Here's how the part is built. I have some questions about the finished solid (model axes, mm). Round coordinates to 2 decimals unless told otherwise and drop trailing zeros. Loops run counter-clockwise (first coordinate to the right, second up) from the corner with the lowest first, then second, coordinate; pieces in that order, holes last. Notation, with made-up numbers: (-39.5, 40.25) - (8.5, 40.25) arc R13 cw to (8.5, 54.25) - close; hole circle Ø5 at (34, -38). An arc over 180 degrees is marked (long way). Answer as a JSON object with one key per item and string values. Group by question number.
1) If I drill on line 1 along Y through (x, z) = (-1, 1.65); line 2 along X through (y, z) = (-53.5, 1.85); line 3 along X through (y, z) = (14.5, 0.5), over which ranges is the centre line in solid material (lowest first)? Write a range as [from, to].
2) I want a section at B-B, the plane x = 38. Please give me the cut outline in (y, z).
3) I want a section at C-C, the plane y = -53.5. Please give me the cut outline in (x, z).
4) I want a section at A-A, the plane z = 1.85. Please give me the cut outline in (x, y), then the cut area to 3 significant figures.
from build123d import *

# Parameters (mm, degrees)
F1_DEPTH    = 2.4268273264
F2_T1_DEPTH = 99.1532575298
F3_T1_DEPTH = 59.396472342
F4_T1_DEPTH = 59.396472342
F5_T1_DEPTH = 107.0840707021
F6_T1_DEPTH = 101.9910508867


# Not quite as in the source:
# - a fillet or chamfer that OpenCascade refuses, or shapes differently, is made with other operations: its cross-section is extruded or revolved along the edge and cut away or added


with BuildPart() as f1:
    # F0 (on Top) → F1 (new body)
    with BuildSketch(Plane.XY):
        Polygon((0, 32.5707793236), (-36.5124791861, 32.5707793236), (-58.7103962898, 0), (0, -63.0669593811), align=None)
        Polygon((36.5124791861, 32.5707793236), (0, 32.5707793236), (0, -63.0669593811), (58.7103962898, 0), align=None)
    extrude(amount=F1_DEPTH)

    # F2: chamfer of 5.08 on 1 edges, made by hand

    # F2_s2 → F2_t1 (cut)
    with BuildSketch(Plane.YZ.offset(-49.5766287649)):
        Polygon((32.5707793236, -2.6531726736), (27.4907793236, 2.4268273264), (32.5707793236, 2.4268273264), align=None)
    extrude(amount=F2_T1_DEPTH, mode=Mode.SUBTRACT)

    # F3: chamfer of 5.08 on 1 edges, made by hand

    # F3_s2 → F3_t1 (cut)
    with BuildSketch(Plane(origin=(7.4722902543, 10.964015938, 0), x_dir=(0, 0, 1), z_dir=(-0.5631734509, -0.8263387103, 0))):
        Polygon((-2.6531726736, 48.5146731522), (2.4268273264, 43.4346731522), (2.4268273264, 48.5146731522), align=None)
    extrude(amount=F3_T1_DEPTH, mode=Mode.SUBTRACT)

    # F4: chamfer of 5.08 on 1 edges, made by hand

    # F4_s2 → F4_t1 (cut)
    with BuildSketch(Plane(origin=(25.9782260477, -38.1175884143, 0), x_dir=(0, 0, 1), z_dir=(-0.5631734509, 0.8263387103, 0))):
        Polygon((-2.6531726736, 48.5146731522), (2.4268273264, 43.4346731522), (2.4268273264, 48.5146731522), align=None)
    extrude(amount=F4_T1_DEPTH, mode=Mode.SUBTRACT)

    # F5: chamfer of 5.08 on 1 edges, made by hand

    # F5_s2 → F5_t1 (cut)
    with BuildSketch(Plane(origin=(-40.354442867, -43.3489155239, 0), x_dir=(0, 0, 1), z_dir=(0.6813742779, 0.7319351703, 0))):
        Polygon((-2.6531726736, 42.9722039049), (2.4268273264, 37.8922039049), (2.4268273264, 42.9722039049), align=None)
    extrude(amount=F5_T1_DEPTH, mode=Mode.SUBTRACT)

    # F6: chamfer of 5.08 on 1 edges, made by hand

    # F6_s2 → F6_t1 (cut)
    with BuildSketch(Plane(origin=(-32.6098884775, 35.0296819984, 0), x_dir=(0, 0, 1), z_dir=(0.6813742779, -0.7319351703, 0))):
        Polygon((-2.6531726736, 42.9722039049), (2.4268273264, 37.8922039049), (2.4268273264, 42.9722039049), align=None)
    extrude(amount=F6_T1_DEPTH, mode=Mode.SUBTRACT)


solid = f1.part
Outcome:
{
 "1": {"line 1": "[-55.68, 28.27]", "line 2": "[-2.75, 2.75]", "line 3": "[-45.01, 45.01]"},
 "2": {"outline": "(-18.35, 0) - (25.68, 0) - (21.37, 2.43) - (-14.79, 2.43) - close"},
 "3": {"outline": "(-5.28, 0) - (5.28, 0) - (1.97, 2.43) - (-1.97, 2.43) - close"},
 "4": {"outline": "(-52.96, 0.44) - (0, -56.46) - (52.96, 0.44) - (34.13, 28.07) - (-34.13, 28.07) - close", "area": "5,420 mm^2"}
}
